```python
from build123d import *

# Parameters (mm, degrees)
CROQUIS1_R              = 8.5
SALIENTE_EXTRUIR1_DEPTH = 5.5
CROQUIS3_R              = 2.85
CORTAR_EXTRUIR1_DEPTH   = 1.2
CROQUIS4_R              = 1.25
CORTAR_EXTRUIR2_DEPTH   = 14.219304066
CROQUIS5_R              = 2.32
CORTAR_EXTRUIR3_DEPTH   = 2.7


with BuildPart() as part:
    # Croquis1 → Saliente-Extruir1 (new body)
    with BuildSketch(Plane.XY):
        Circle(CROQUIS1_R)
    extrude(amount=SALIENTE_EXTRUIR1_DEPTH)

    # Croquis2 → Cortar-Revolución1 (revolve, cut)
    with BuildSketch(Plane(origin=(0, 0, 0), x_dir=(0, 0, -1), z_dir=(1, 0, 0)), mode=Mode.PRIVATE) as cortar_revoluci_n1_sk:
        Polygon((-5.5, 8.5), (-4.25, 8.5), (-4.25, 5.5), (-1.25, 5.5), (-1.25, 8.5), (0, 8.5), (0, 8.952172256), (-5.5, 8.952172256), align=None)
    revolve(cortar_revoluci_n1_sk.sketch.rotate(Axis((0, 0, 0), (0, 0, 1)), 90), axis=Axis((0, 0, 0), (0, 0, 1)), mode=Mode.SUBTRACT)

    # Croquis3 → Cortar-Extruir1 (cut)
    with BuildSketch(Plane.XY.offset(5.5)):
        Circle(CROQUIS3_R)
    extrude(amount=-CORTAR_EXTRUIR1_DEPTH, mode=Mode.SUBTRACT)

    # Croquis4 → Cortar-Extruir2 (cut, through all)
    with BuildSketch(Plane.XY.offset(5.5)):
        Circle(CROQUIS4_R)
    extrude(amount=-CORTAR_EXTRUIR2_DEPTH, mode=Mode.SUBTRACT)

    # Croquis5 → Cortar-Extruir3 (cut)
    with BuildSketch(Plane(origin=(0, 0, 0), x_dir=(-1, 0, 0), z_dir=(0, 0, -1))):
        Circle(CROQUIS5_R)
    extrude(amount=-CORTAR_EXTRUIR3_DEPTH, mode=Mode.SUBTRACT)


solid = part.part
```
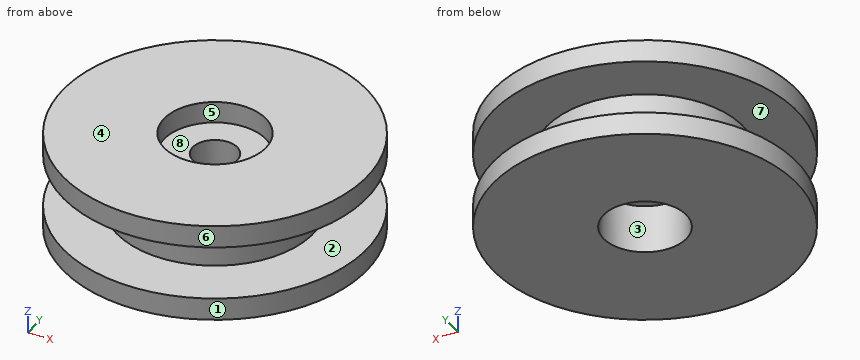
Build history of the part. All positions in model axes, mm. Face numbers are marked on the shaded views. A direction names the side the tool comes from. Round coordinates to 2 decimals unless told otherwise and drop trailing zeros. Write each loop counter-clockwise with the first axis right and the second up, starting at its lowest first coordinate (ties: lowest second). Pieces come first, ordered by that corner, then holes. Notation, with made-up numbers: (84, 21.25) - (111, 21.25) arc R5 ccw to (111, 30.25) - close; hole circle Ø11 at (-31.75, 45). An arc over 180 degrees is marked (long way). Write each question's results on one line, items separated by ' | '. Start each with the question number.
Item 1: Wall check: L1, parallel to Y at x = 0, z = 0.75; L2, parallel to Z at x = -0.25, y = 6; L3, parallel to Y at x = 0, z = 5.1. Give the ranges that are in metal, low to high. Write a range as [from, to].
Item 2: Saw through at C-C (z = 1.7). Write the cut outline in (x, y), and give its area (3 significant figures).
Item 3: Saw through at A-A (y = 7.5). Write the cut outline in (x, z), and give its area (3 significant figures).
Item 4: Which spindle directions (+Z, -Z, +X, -X, +Y, -Y) get a long thin tool onto all of the face, cutting with end or side? Do the marked faces 1, 2, 3, 4 and 5. Say none if no direction does.
Item 5: Saw through at B-B (x = 0). Write the cut outline in (y, z).
Item 6: Mould opens along X. For the marked faces 6, 7 and 8 say: pulls with the +X half, pulls with the -X half, needs draft (parallel to the pull), parting line crosses it, or undercut.
Item 7: Drop flat-ended pins along their axis: P1, Ø3.5, axis at x = 0, y = 0, coming from the -Z side; P2, Ø1, axis at y = -1.5, z = 2.5, coming from the +X side; P3, Ø2, axis at x = 0, y = 0, coming from the +Z side. Give the stop position or say it passes through.
Results are:
1) L1: y = [-8.5, -2.32], [2.32, 8.5] | L2: z = [0, 1.25], [4.25, 5.5] | L3: y = [-8.5, -2.85], [2.85, 8.5]
2) outline: circle Ø11 at (0, 0); hole circle Ø4.64 at (0, 0) | area: 78.1 mm²
3) outline: (-4, 0) - (4, 0) - (4, 1.25) - (-4, 1.25) - close; (-4, 4.25) - (4, 4.25) - (4, 5.5) - (-4, 5.5) - close | area: 20.0 mm²
4) face 1: +Z, -Z | face 2: none | face 3: -Z | face 4: +Z, +X, -X, +Y, -Y | face 5: +Z
5) outline: (-8.5, 0) - (-2.32, 0) - (-2.32, 2.7) - (-1.25, 2.7) - (-1.25, 4.3) - (-2.85, 4.3) - (-2.85, 5.5) - (-8.5, 5.5) - (-8.5, 4.25) - (-5.5, 4.25) - (-5.5, 1.25) - (-8.5, 1.25) - close; (1.25, 2.7) - (2.32, 2.7) - (2.32, 0) - (8.5, 0) - (8.5, 1.25) - (5.5, 1.25) - (5.5, 4.25) - (8.5, 4.25) - (8.5, 5.5) - (2.85, 5.5) - (2.85, 4.3) - (1.25, 4.3) - close
6) face 6: parting line crosses it | face 7: needs draft | face 8: undercut
7) P1: stops at z = 2.7 | P2: stops at x = 5.41 | P3: passes through
